from build123d import *

# Parameters (mm, degrees)
F0_W      = 44
F0_H      = 144
F0_W_2    = 40
F0_H_2    = 140
F1_DEPTH  = 2
F2_DEPTH  = 25
F5_DEPTH  = 2
F6_DEPTH  = 2
F7_DEPTH  = 5
F8_DEPTH  = 4
F10_DEPTH = 32.0010001
F9_W      = 36
F9_H      = 2
F9_W_2    = 2
F9_H_2    = 73
F11_DEPTH = 1
F12_R     = 1.99999


# Not quite as in the source:
# - a fillet or chamfer is up to 0.001 mm smaller than in the source, because OpenCascade refuses the exact size


with BuildPart() as f1:
    # F0 (on Top) → F1 (new body)
    with BuildSketch(Plane.XY):
        Rectangle(F0_W, F0_H)
        Rectangle(F0_W_2, F0_H_2, mode=Mode.SUBTRACT)
        Rectangle(F0_W_2, F0_H_2)
    extrude(amount=-F1_DEPTH)

    # F0 (on Top) → F2 (join)
    with BuildSketch(Plane.XY):
        Rectangle(F0_W, F0_H)
        Rectangle(F0_W_2, F0_H_2, mode=Mode.SUBTRACT)
    extrude(amount=F2_DEPTH)

    # F3 (on face) → F5 (join)
    with BuildSketch(Plane.YZ.offset(22)):
        with BuildLine():
            add(Edge.make_bspline(
                [(4.7271151019, 25), (15.348527654, 25.1268953042), (37.9929862917, 27.4159301893), (60.2495129104, 28.4605212291), (72, 29)],
                knots=[0.5326300299, 0.5326300299, 0.5326300299, 0.5326300299, 0.7517880542, 1, 1, 1, 1], degree=3))
            Line((4.7271151019, 25), (72, 25))
            Line((72, 25), (72, 29))
        make_face()
        with BuildLine():
            Line((-72, 30), (-72, 25))
            Line((-72, 25), (0.6763282883, 25))
            add(Edge.make_bspline(
                [(-72, 30), (-60.2445668251, 29.5430569498), (-36.4192696174, 28.5876982607), (-11.9822251211, 25.1864507884), (0.4508819142, 25.0028330974), (0.6763282883, 25)],
                knots=[0, 0, 0, 0, 0.2482119458, 0.5001170824, 0.504769099, 0.504769099, 0.504769099, 0.504769099], degree=3))
        make_face()
    extrude(amount=-F5_DEPTH)

    # F4 (on face) → F6 (join)
    with BuildSketch(Plane(origin=(-22, 0, 0), x_dir=(0, -1, 0), z_dir=(-1, 0, 0))):
        with BuildLine():
            Line((-72, 29), (-72, 25))
            Line((-72, 25), (-4.7271151019, 25))
            add(Edge.make_bspline(
                [(-72, 29), (-60.2495129104, 28.4605212291), (-37.9929862917, 27.4159301893), (-15.348527654, 25.1268953042), (-4.7271151019, 25)],
                knots=[0, 0, 0, 0, 0.2482119458, 0.4673699701, 0.4673699701, 0.4673699701, 0.4673699701], degree=3))
        make_face()
        with BuildLine():
            Line((0, 25), (72, 25))
            Line((72, 25), (72, 30))
            add(Edge.make_bspline(
                [(0, 25.01), (12.2074400514, 25.2177971205), (36.4192696174, 28.5876982607), (60.2445668251, 29.5430569498), (72, 30)],
                knots=[0.4998829176, 0.4998829176, 0.4998829176, 0.4998829176, 0.7517880542, 1, 1, 1, 1], degree=3))
            Line((0, 25.01), (0, 25))
        make_face()
    extrude(amount=-F6_DEPTH)

    # F7 (add): a face of the model
    f7_faces = [f1.faces().sort_by_distance(p)[0] for p in [
        (0, -71, 25),
    ]]
    extrude(f7_faces, amount=F7_DEPTH)

    # F8 (add): a face of the model
    f8_faces = [f1.faces().sort_by_distance(p)[0] for p in [
        (0, 71, 25),
    ]]
    extrude(f8_faces, amount=F8_DEPTH)

    # F9 (on face) → F10 (cut, through all)
    with BuildSketch(Plane(origin=(0, 0, -2), x_dir=(1, 0, 0), z_dir=(0, 0, -1))):
        Polygon((20, 35.5240486562), (20, 60.5240486562), (-20, 60.5240486562), (-20, 35.5240486562), (-18, 35.5240486562), (-18, -37.4759513438), (18, -37.4759513438), (18, 35.5240486562), align=None)
    extrude(amount=-F10_DEPTH, mode=Mode.SUBTRACT)

    # F9 (on face) → F11 (cut)
    with BuildSketch(Plane(origin=(0, 0, -2), x_dir=(1, 0, 0), z_dir=(0, 0, -1))):
        with Locations((0, -38.4759513438)):
            Rectangle(F9_W, F9_H)
        with Locations((-19, -38.4759513438)):
            Rectangle(F9_W_2, F9_H)
        with Locations((-19, -0.9759513438)):
            Rectangle(F9_W_2, F9_H_2)
        with Locations((19, -38.4759513438)):
            Rectangle(F9_W_2, F9_H)
        with Locations((19, -0.9759513438)):
            Rectangle(F9_W_2, F9_H_2)
    extrude(amount=-F11_DEPTH, mode=Mode.SUBTRACT)

    # F12 (radius 2 in the source; OpenCascade refuses exactly that, so slightly less here)
    f12_edges = [f1.edges().sort_by_distance(p)[0] for p in [
        (0, -72, -2),
        (-22, 0, -2),
        (22, 0, -2),
        (-22, -72, 14),
        (22, -72, 14),
        (0, 72, -2),
        (-22, 72, 13.5),
        (22, 72, 13.5),
    ]]
    fillet(f12_edges, radius=F12_R)


solid = f1.part
For this review, take the finished solid that the model builds, in its own axes (mm). A direction names the side the tool comes from. Round coordinates to 2 decimals unless told otherwise and drop trailing zeros. Loops run counter-clockwise (first coordinate to the right, second up) from the corner with the lowest first, then second, coordinate; pieces in that order, holes last. Notation, with made-up numbers: (-6.5, 86) - (11.5, 86) arc R22 cw to (11.5, 117) - close; hole circle Ø5 at (50, 41.25). An arc over 180 degrees is marked (long way). One line per question, with ' | ' between items.
Q1. For pin 1 (2 mm diameter, centred on x = -9.5, z = -1, fed in from +Y); pin 2 (2 mm diameter, centred on x = -21, y = 2, fed in from +Z); pin 3 (3 mm diameter, centred on x = -9, y = -64, fed in from +Z); pin 4 (0.8 mm diameter, centred on x = 19.5, z = -0.5, fed in from -Y), all flat-tipped, find the tip position at first contact; note any pin that passes through.
Taken from the geometry:
pin 1: stops at y = 72 | pin 2: stops at z = 25 | pin 3: stops at z = 0 | pin 4: stops at y = -72
Q2. Tool access review of faces 4 (the flat face through (0, -70, 15)), 5 (the flat face through (19, 13, -1)), 6 (the flat face through (0, 72, 14)): name each direction out of +Z, -Z, +X, -X, +Y, -Y from which nothing blocks a thin tool from reaching the whole face with its end or side.
Taken from the geometry:
face 4: +Z | face 5: -Z | face 6: +Z, -Z, +X, -X, +Y
Q3. Take a section at B-B (z = 10.5). Give the boundary of the cut face in (x, y).
Taken from the geometry:
outline: (-22, -70) arc R2 ccw to (-20, -72) - (20, -72) arc R2 ccw to (22, -70) - (22, 70) arc R2 ccw to (20, 72) - (-20, 72) arc R2 ccw to (-22, 70) - close; hole (-20, -70) - (20, -70) - (20, 70) - (-20, 70) - close
Q4. Take a section at A-A (x = 7). Give the boundary of the cut face in (y, z).
Taken from the geometry:
outline: (-72, 0) arc R2 ccw to (-70, -2) - (-60.52, -2) - (-60.52, 0) - (-70, 0) - (-70, 30) - (-72, 30) - close; (37.48, -1) - (39.48, -1) - (39.48, -2) - (70, -2) arc R2 ccw to (72, 0) - (72, 29) - (70, 29) - (70, 0) - (37.48, 0) - close
Q5. For line 1 along Y through (x, z) = (17.5, 10); line 2 along X through (y, z) = (-12.5, 22.5); line 3 along Z through (x, y) = (1, 44), list the stretches that pass through material, from the lowest coordinate up. Write a range as [from, to].
Taken from the geometry:
line 1: y = [-72, -70], [70, 72] | line 2: x = [-22, -20], [20, 22] | line 3: z = [-2, 0]
Q6. The part is to be moulded in two halves that separate along X. For faces 1 (the flat face through (22, 1, 15)), 2 (the flat face through (20, 1, 14)), 3 (the flat face through (0, -72, 15)), say which applies: released by +X, released by -X, zero draft, split by the parting line, or undercut.
Taken from the geometry:
face 1: released by +X | face 2: undercut | face 3: zero draft
